from build123d import *

# Parameters (mm, degrees)
SKETCH1_W                       = 80
SKETCH1_H                       = 10
BOSS_EXTRUDE1_DEPTH             = 120
SKETCH2_R                       = 14.2875
HOLES_DEPTH                     = 127
SKETCH5_W                       = 16.58
SKETCH5_H                       = 240
WEDGE_SHAPE_DEPTH               = 127.885775404
FILLET6_START                   = -6
FILLET6_DEPTH                   = 12
TAP_DRILL_FOR_M6X1_0_TAP1_D     = 5
TAP_DRILL_FOR_M6X1_0_TAP1_DEPTH = 8.651


with BuildPart() as part:
    # Sketch1 → Boss-Extrude1 (new, symmetric)
    with BuildSketch(Plane(origin=(0, 0, 0), x_dir=(1, 0, 0), z_dir=(0, 1, 0))):
        Rectangle(SKETCH1_W, SKETCH1_H)
    extrude(amount=BOSS_EXTRUDE1_DEPTH, both=True)

    # Sketch2 → Holes (cut)
    with BuildSketch(Plane.XY.offset(5)):
        with Locations((0, -95.26)):
            Circle(SKETCH2_R)
        Polygon((3.666174209, 98.65), (7.332348419, 105), (3.666174209, 111.35), (-3.666174209, 111.35), (-7.332348419, 105), (-3.666174209, 98.65), align=None)
    extrude(amount=-HOLES_DEPTH, mode=Mode.SUBTRACT)

    # Sketch5 → Wedge shape (cut, through all)
    with BuildSketch(Plane(origin=(0, 0, -5), x_dir=(-1, 0, 0), z_dir=(0, 0, -1))):
        with BuildLine():
            Line((40, 104.109763944), (21.447331521, -120))
            ThreePointArc((21.447331521, -120), (30.723665761, -120.383309719), (40, -120))
            Line((40, -120), (40, 104.109763944))
        make_face()
        with Locations((-31.71, 0)):
            Rectangle(SKETCH5_W, SKETCH5_H)
    extrude(amount=-WEDGE_SHAPE_DEPTH, mode=Mode.SUBTRACT)

    # Fillet6: read off the stored shape, not the designer's step
    # Fillet6 outline → Fillet6 (cut)
    with BuildSketch(Plane.XY.offset(FILLET6_START)):
        with BuildLine():
            ThreePointArc((-0.005704702, -119.950382649), (-15.93515227, -112.84990156), (-23.346182643, -97.062540783))
            Line((-23.346182643, -97.062540783), (-21.447331521, -120))
            Line((-21.447331521, -120), (23.42, -120))
            Line((23.42, -120), (23.42, -95))
            ThreePointArc((23.42, -95), (16.645769976, -112.112022346), (-0.005704702, -119.950382649))
        make_face()
        with BuildLine():
            Line((-40, 104.109763944), (-39.075113631, 92.937459217))
            ThreePointArc((-39.075113631, 92.937459217), (-32.552777964, 111.932756427), (-14.160340393, 120))
            Line((-14.160340393, 120), (-40, 120))
            Line((-40, 120), (-40, 104.109763944))
        make_face()
        with BuildLine():
            ThreePointArc((-1.58, 120), (16.09766953, 112.67766953), (23.42, 95))
            Line((23.42, 95), (23.42, 120))
            Line((23.42, 120), (-1.58, 120))
        make_face()
    extrude(amount=FILLET6_DEPTH, mode=Mode.SUBTRACT)

    # Tap Drill for M6x1.0 Tap1
    with Locations(Plane(origin=(0, 120, -0.37225415), x_dir=(0, 0, 1), z_dir=(0, 1, 0))):
        with Locations((0, 0)):
            Hole(TAP_DRILL_FOR_M6X1_0_TAP1_D / 2, depth=TAP_DRILL_FOR_M6X1_0_TAP1_DEPTH)


solid = part.part
Verification items for the finished model (mm, model axes). A direction names the side the tool comes from. Coordinates: 2 decimals unless noted, no trailing zeros. Loops run counter-clockwise (first coordinate to the right, second up) from the corner with the lowest first, then second, coordinate; pieces in that order, holes last. Notation, with made-up numbers: (47, 13) -> (76, 13) arc R20 cw to (76, 41) -> close; hole circle Ø4 at (0.25, 84.5). An arc over 180 degrees is marked (long way). Answer as a JSON object with one key per item and string values. Group by question number.
Item 1: Mould release check, pull along Y, two halves, no side actions. Record for faces 1 (the cylindrical face through (16.825, -111.919, -0.07)), 2 (the flat face through (-1, 2, -5)), 3 (the flat face through (5.525, 108.131, 0.07)): +Y half, -Y half, draft (parallel to the pull), parting line (faces both ways), or undercut.
Item 2: Sectioned sample at A-A on x = -11. Record the boundary of the cut face in (y, z).
Item 3: Tool access check on faces 4 (the cylindrical face through (-1.521, 115.614, 1.612)), 5 (the flat face through (-1, 2, 5)), 6 (the flat face through (-5.525, 101.869, 0.07)). Record the directions out of +Z, -Z, +X, -X, +Y, -Y that give a thin tool (end or side, any length) a straight path to the whole face; none if there is none.
Item 4: Depth check by flat-ended pin: pin 1 (2 mm diameter, centred on x = -0.5, z = -2.5, fed in from -Y); pin 2 (2 mm diameter, centred on x = -1, z = -0.5, fed in from +Y); pin 3 (3 mm diameter, centred on x = -28, z = -1, fed in from +Y); pin 4 (1.5 mm diameter, centred on x = 3, z = -2.5, fed in from -Y). Enter the tip coordinate at first touch or a pass-through.
Item 5: Scan lines: probe 1 along Y at (x, z) = (0, 1.75); probe 2 along Y at (x, z) = (6.5, -4); probe 3 along Z at (x, y) = (0, 114.25). Record each from-to range of solid material in increasing order.
Item 6: Sectioned sample at D-D on x = 17. Record the boundary of the cut face in (y, z).
Item 7: Sectioned sample at C-C on y = -76.5. Record the boundary of the cut face in (x, z), plus the area to 3 significant figures.
Evaluation:
{
 "1": {"face 1": "-Y half", "face 2": "draft", "face 3": "undercut"},
 "2": {"outline": "(-116.61, -5) -> (-104.38, -5) -> (-104.38, 5) -> (-116.61, 5) -> close; (-86.14, -5) -> (120, -5) -> (120, 5) -> (-86.14, 5) -> close"},
 "3": {"face 4": "+Y", "face 5": "+Z, +X, -X, +Y, -Y", "face 6": "+Z, -Z"},
 "4": {"pin 1": "stops at y = -119.95", "pin 2": "stops at y = 98.65", "pin 3": "stops at y = 116.74", "pin 4": "stops at y = -119.7"},
 "5": {"probe 1": "y = -119.95 to -109.55, -80.97 to 98.65", "probe 2": "y = -118.66 to -107.98, -82.54 to 103.56, 106.44 to 118.66", "probe 3": "z = -5 to -2.87, 2.13 to 5"},
 "6": {"outline": "(-111.73, -5) -> (111.73, -5) -> (111.73, 5) -> (-111.73, 5) -> close"},
 "7": {"outline": "(-25.05, -5) -> (23.42, -5) -> (23.42, 5) -> (-25.05, 5) -> close", "area": "485 mm²"}
}
